Design review of the part shown in the three views and the two pictorial views. Dimensions are in mm from the part's minimum x, y and z. A direction names the side the tool comes from. Round coordinates to 2 decimals unless told otherwise and drop trailing zeros. Loops run counter-clockwise (first coordinate to the right, second up) from the corner with the lowest first, then second, coordinate; pieces in that order, holes last. Notation, with made-up numbers: (42, -29) -> (82, -29) arc R26 cw to (82, -13) -> close; hole circle Ø1 at (-1, 69.5). An arc over 180 degrees is marked (long way). Return JSON: item names as keys, results as strings. Group by question number.
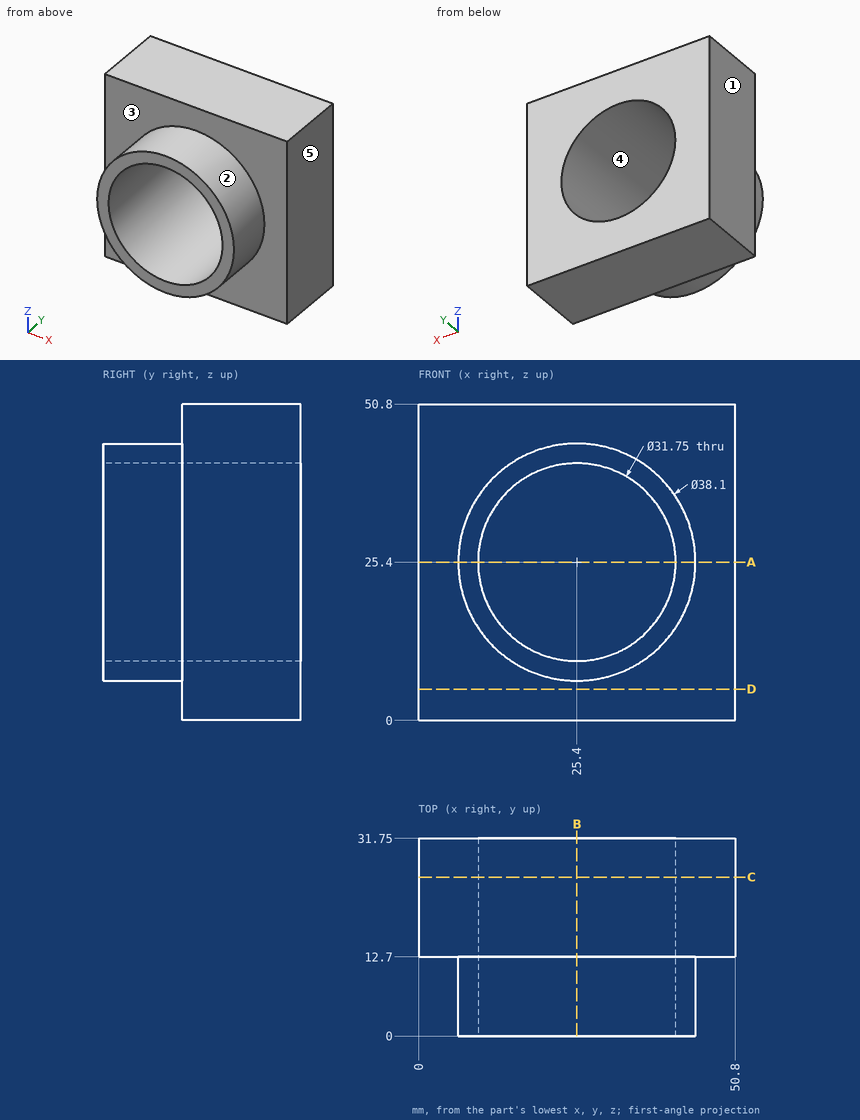
1. We need section A-A, the plane z = 25.4. Write out the cut boundary in (x, y) (3 decimals).
2. Tool access review of the marked faces 1 and 2: name each direction out of +Z, -Z, +X, -X, +Y, -Y from which nothing blocks a thin tool from reaching the whole face with its end or side.
3. We need section B-B, the plane x = 25.4. Write out the cut boundary in (y, z) (3 decimals).
4. For P1, Ø3, axis at y = 7.5, z = 23.5, coming from the +X side; P2, Ø19, axis at x = 25.4, z = 25.4, coming from the +Y side; P3, Ø4, axis at y = 5, z = 35, coming from the -X side; P4, Ø4, axis at y = 12.5, z = 33, coming from the +X side, all flat-tipped, find the tip position at first contact; note any pin that passes through.
5. We need section C-C, the plane y = 25.5. Write out the cut boundary in (x, z) (3 decimals), then the cut area to 3 significant figures.
6. Wall thickness on line 1 (Z direction, x = 25.4, y = 23.5) (3 decimals); line 2 (X direction, y = 13, z = 25); line 3 (Y direction, x = 42, z = 47): over which ranges is each line inside the solid? List them lowest first.
7. Draft analysis for pull direction X (two halves, no side actions). For the marked faces 3, 4 and 5, state which applies: pulls with the +X half, pulls with the -X half, needs draft (parallel to the pull), parting line crosses it, or undercut.
8. We need section D-D, the plane z = 5. Write out the cut boundary in (x, y), then the cut area to 3 significant figures.
Check sheet entries:
{
 "1": {"outline": "(0, 12.7) -> (6.35, 12.7) -> (6.35, 0) -> (9.525, 0) -> (9.525, 31.75) -> (0, 31.75) -> close; (41.275, 0) -> (44.45, 0) -> (44.45, 12.7) -> (50.8, 12.7) -> (50.8, 31.75) -> (41.275, 31.75) -> close"},
 "2": {"face 1": "+Z, -Z, -X, +Y, -Y", "face 2": "-Y"},
 "3": {"outline": "(0, 6.35) -> (12.7, 6.35) -> (12.7, 0) -> (31.75, 0) -> (31.75, 9.525) -> (0, 9.525) -> close; (0, 41.275) -> (31.75, 41.275) -> (31.75, 50.8) -> (12.7, 50.8) -> (12.7, 44.45) -> (0, 44.45) -> close"},
 "4": {"P1": "stops at x = 44.45", "P2": "passes through", "P3": "stops at x = 7.93", "P4": "stops at x = 50.8"},
 "5": {"outline": "(0, 0) -> (50.8, 0) -> (50.8, 50.8) -> (0, 50.8) -> close; hole circle Ø31.75 at (25.4, 25.4)", "area": "1,790 mm²"},
 "6": {"line 1": "z = 0 to 9.525, 41.275 to 50.8", "line 2": "x = 0 to 9.53, 41.27 to 50.8", "line 3": "y = 12.7 to 31.75"},
 "7": {"face 3": "needs draft", "face 4": "undercut", "face 5": "pulls with the +X half"},
 "8": {"outline": "(0, 12.7) -> (50.8, 12.7) -> (50.8, 31.75) -> (0, 31.75) -> close", "area": "968 mm²"}
}
